Read the model definition and answer for the solid it produces. Units are mm, in the model's axes. A direction names the side the tool comes from. Coordinates: 2 decimals unless noted, no trailing zeros. Loops run counter-clockwise (first coordinate to the right, second up) from the corner with the lowest first, then second, coordinate; pieces in that order, holes last.
Q1. Section B-B (z = 6.25) is taken. Give the vertices of the cut face in (x, y).
Q2. Which of the six approach directions +Z, -Z, +X, -X, +Y, -Y give full straight-line access (tool end or side, diameter ignored) to faces 5 (the face through (3.21, 1.94, 2.56)), 6 (the face through (-3, 0, 7.1)), 7 (the face through (-5.44, -3.08, 0.74))?
Q3. Section D-D (y = -4.5) is taken. Give the vertices of the cut face in (x, z).
Q4. Flat-ended cylindrical pins translate along their axes: P1, Ø2, axis at y = -1.5, z = 9.5, coming from the -X side; P2, Ø1, axis at x = -1, y = -4.5, coming from the -Z side; P3, Ø4, axis at x = 0, y = 0, coming from the -Z side; P4, Ø4, axis at y = -2.5, z = 11.5, coming from the -X side. Find the tip coordinate at first contact, or state that the pin passes through.
Q5. Straight lines are drawn through the part: line 1 (Z direction, x = -5.5, y = -2); line 2 (Z direction, x = 3.5, y = -5); line 3 (Y direction, x = 0, z = 4.6). For each, find the intervals that lie inside material, in ascending order.
Q6. Section C-C (x = -1.5) is taken. Give the vertices of the cut face in (y, z).
Q7. The mould has two halves that part along X. Classify faces 1 (the face through (3.448, -2.028, 9.077)), 2 (the face through (0, -6.25, 9)), 3 (the face through (5.44, 3.08, 6.9)), 4 (the face through (-0.54, -2.44, 5.33)): pulls with the +X half, pulls with the -X half, needs draft (parallel to the pull), parting line crosses it, or undercut.
Q8. Section A-A (x = -3) is taken. Give the vertices of the cut face in (y, z), then the cut area to 3 significant figures.
from build123d import *

# Parameters (mm, degrees)
F0_R     = 2.5
F1_DEPTH = 14
F2_W     = 17.4719977542
F2_H     = 2.1
F3_DEPTH = 10
F5_START = -3
F5_DEPTH = 3.9


with BuildPart() as f1:
    # F0 (on Top) → F1 (new body)
    with BuildSketch(Plane.XY):
        Polygon((-3.6084391824, -6.25), (3.6084391824, -6.25), (7.2168783649, 0), (3.6084391824, 6.25), (-3.6084391824, 6.25), (-7.2168783649, 0), align=None)
        Circle(F0_R, mode=Mode.SUBTRACT)
    extrude(amount=F1_DEPTH)

    # F2 (on face) → F3 (cut)
    with BuildSketch(Plane(origin=(-5.4126587737, -3.125, 0), x_dir=(0.5, -0.8660254038, 0), z_dir=(-0.8660254038, -0.5, 0))):
        with Locations((0, 2.55)):
            Rectangle(F2_W, F2_H)
    extrude(amount=-F3_DEPTH, mode=Mode.SUBTRACT)

    # F4 (on face) → F5 (cut)
    with BuildSketch(Plane.XY.offset(14).offset(F5_START)):
        Polygon((2.3094010768, 4), (-2.3094010768, 4), (-10.6891589239, 4), (-10.3349462152, -4), (-2.3094010768, -4), (2.3094010768, -4), (4.6188021535, 0), align=None)
    extrude(amount=-F5_DEPTH, mode=Mode.SUBTRACT)


solid = f1.part
Numbers:
1. outline: (-7.22, 0) - (-3.61, -6.25) - (3.61, -6.25) - (7.22, 0) - (3.61, 6.25) - (-3.61, 6.25) - close; hole circle Ø5 at (0, 0)
2. face 5: -X, -Y
2. face 6: -X
2. face 7: +Z, -Z, -X, -Y
3. outline: (-4.62, 0) - (4.62, 0) - (4.62, 1.5) - (-4.62, 1.5) - close; (-4.62, 3.6) - (4.62, 3.6) - (4.62, 14) - (-4.62, 14) - close
4. P1: stops at x = 3.18
4. P2: stops at z = 0
4. P3: passes through
4. P4: stops at x = -6.93
5. line 1: z = 0 to 1.5, 3.6 to 7.1, 11 to 14
5. line 2: z = 0 to 1.5, 3.6 to 14
5. line 3: y = -6.25 to -2.5, 2.5 to 6.25
6. outline: (-6.25, 0) - (-2, 0) - (-2, 1.5) - (-6.25, 1.5) - close; (-6.25, 3.6) - (-2, 3.6) - (-2, 7.1) - (-4, 7.1) - (-4, 11) - (-2, 11) - (-2, 14) - (-6.25, 14) - close; (2, 0) - (6.25, 0) - (6.25, 1.5) - (2, 1.5) - close; (2, 3.6) - (6.25, 3.6) - (6.25, 14) - (2, 14) - (2, 11) - (4, 11) - (4, 7.1) - (2, 7.1) - close
7. face 1: pulls with the -X half
7. face 2: needs draft
7. face 3: pulls with the +X half
7. face 4: undercut
8. outline: (-6.25, 0) - (6.25, 0) - (6.25, 1.5) - (-6.25, 1.5) - close; (-6.25, 3.6) - (6.25, 3.6) - (6.25, 14) - (-6.25, 14) - close; hole (-4, 7.1) - (4, 7.1) - (4, 11) - (-4, 11) - close
8. area: 118 mm2
